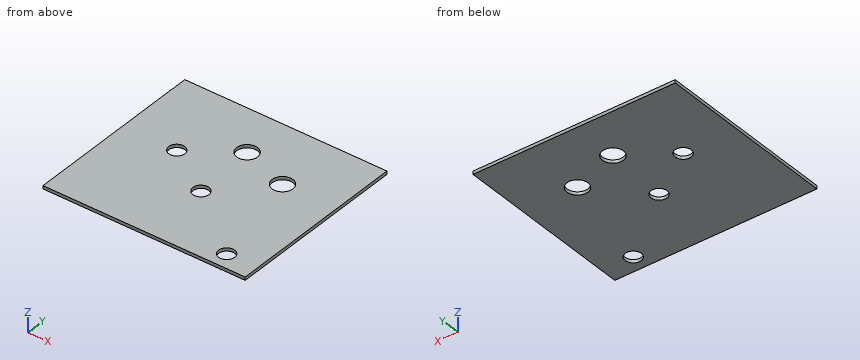
```python
from build123d import *

# Parameters (mm, degrees)
SKETCH1_W                               = 125.870370198
SKETCH1_H                               = 113.481751874
BOSS_EXTRUDE1_DEPTH                     = 2
CBORE_FOR_M5_HEX_HEAD_BOLT1_D           = 5.5
CBORE_FOR_M5_HEX_HEAD_BOLT1_CBORE_D     = 13
CBORE_FOR_M5_HEX_HEAD_BOLT1_CBORE_DEPTH = 3.5
SKETCH4_R                               = 5
CUT_EXTRUDE1_DEPTH                      = 2


with BuildPart() as part:
    # Sketch1 → Boss-Extrude1 (new body)
    with BuildSketch(Plane.XY):
        with Locations((-62.935185099, 56.740875937)):
            Rectangle(SKETCH1_W, SKETCH1_H)
    extrude(amount=BOSS_EXTRUDE1_DEPTH)

    # CBORE for M5 Hex Head Bolt1 (through all)
    with Locations(Plane(origin=(0, 0, 0), x_dir=(-1, 0, 0), z_dir=(0, 0, -1))):
        with Locations((33.729629401, 73.217807093), (64.028441194, 83.838009165)):
            CounterBoreHole(CBORE_FOR_M5_HEX_HEAD_BOLT1_D / 2, CBORE_FOR_M5_HEX_HEAD_BOLT1_CBORE_D / 2, CBORE_FOR_M5_HEX_HEAD_BOLT1_CBORE_DEPTH)

    # Sketch4 → Cut-Extrude1 (cut)
    with BuildSketch(Plane(origin=(0, 0, 0), x_dir=(-1, 0, 0), z_dir=(0, 0, -1))):
        with Locations((19.304896116, 10)):
            Circle(SKETCH4_R)
        with Locations((61.810693115, 44.050073834)):
            Circle(SKETCH4_R)
        with Locations((92.396875082, 64.050073834)):
            Circle(SKETCH4_R)
    extrude(amount=-CUT_EXTRUDE1_DEPTH, mode=Mode.SUBTRACT)


solid = part.part
```
Check sheet for the modelled part. Datum: model origin and axes. Units: mm. Coordinates: 2 decimals unless noted, no trailing zeros. Order: outer loops, then holes, each group sorted by start corner. A loop starts at its lowest first (then second) coordinate and runs counter-clockwise, first axis right, second up. Notation, with made-up numbers: (21.5, 46) -> (28.5, 46) arc R17 ccw to (28.5, 51) -> close; hole circle Ø6 at (-18, 75.25). An arc over 180 degrees is marked (long way). Write item = value, one per line. Start each with the question number.
1) Material ranges on L1, parallel to Y at x = -65, z = 1.25; L2, parallel to X at y = 9.5, z = 1.65; L3, parallel to Y at x = -39.5, z = 1, recorded low to high.
2) Cross-section at A-A (y = 10). Enter the section's corners in (x, z), then the cut area to 3 significant figures.
3) Go/stop test with a flat-tipped pin: P1, Ø10.5, axis at x = -33.73, y = 73.22, coming from the -Z side. Record where the tip stops, or that it passes through.
4) Cross-section at C-C (z = 0.55). Enter the section's corners in (x, y).
5) Cross-section at B-B (x = -89.5). Enter the section's corners in (y, z), then the cut area to 3 significant figures.
Ans:
q1.L1 = 0 to 40.2, 47.9 to 77.41, 90.26 to 113.48
q1.L2 = -125.87 to -24.28, -14.33 to 0
q1.L3 = 0 to 70.23, 76.21 to 113.48
q2.outline = (-125.87, 0) -> (-24.3, 0) -> (-24.3, 2) -> (-125.87, 2) -> close; (-14.3, 0) -> (0, 0) -> (0, 2) -> (-14.3, 2) -> close
q2.area = 232 mm²
q3.P1 = through
q4.outline = (-125.87, 0) -> (0, 0) -> (0, 113.48) -> (-125.87, 113.48) -> close; hole circle Ø10 at (-92.4, 64.05); hole circle Ø13 at (-64.03, 83.84); hole circle Ø10 at (-61.81, 44.05); hole circle Ø13 at (-33.73, 73.22); hole circle Ø10 at (-19.3, 10)
q5.outline = (0, 0) -> (59.97, 0) -> (59.97, 2) -> (0, 2) -> close; (68.13, 0) -> (113.48, 0) -> (113.48, 2) -> (68.13, 2) -> close
q5.area = 211 mm²
